Part model, mm, in its own coordinate system. A direction names the side the tool comes from. Round coordinates to 2 decimals unless told otherwise and drop trailing zeros. Order: outer loops, then holes, each group sorted by start corner. A loop starts at its lowest first (then second) coordinate and runs counter-clockwise, first axis right, second up. Notation, with made-up numbers: (66, 46) -> (114, 46) arc R29 ccw to (114, 78) -> close; hole circle Ø4 at (57, 71.5). An arc over 180 degrees is marked (long way). Answer as a JSON object with one key per item and string values. Group by question number.
```python
from build123d import *

# Parameters (mm, degrees)
SKETCH_5_R          = 3
EXTRUDE_4_DEPTH     = 5
CUT_EXTRUDE_2_DEPTH = 8.5
CUT_EXTRUDE_4_DEPTH = 8.5


with BuildPart() as part:
    # Sketch 5 → Extrude 4 (new body)
    with BuildSketch(Plane(origin=(0, 0, 0), x_dir=(1, 0, 0), z_dir=(0, 1, 0))):
        Polygon((-86.043555275, 72.404841583), (-103.043555275, 72.404841583), (-103.043555275, -36.501510282), (78.477843527, -36.501510282), (78.477843527, 72.404841583), (62.047530944, 72.404841583), (62.047530944, -18.742135335), (-86.043555275, -18.742135335), align=None)
        with BuildLine():
            ThreePointArc((-29.666312365, -34.509375465), (-31.566312365, -32.609375465), (-29.666312365, -30.709375465))
            Line((-29.666312365, -30.709375465), (-24.596682227, -30.709375465))
            ThreePointArc((-24.596682227, -30.709375465), (-22.696682227, -32.609375465), (-24.596682227, -34.509375465))
            Line((-24.596682227, -34.509375465), (-29.666312365, -34.509375465))
        make_face(mode=Mode.SUBTRACT)
        with BuildLine():
            ThreePointArc((0.233182571, -34.509375465), (-1.666817429, -32.609375465), (0.233182571, -30.709375465))
            Line((0.233182571, -30.709375465), (5.30281271, -30.709375465))
            ThreePointArc((5.30281271, -30.709375465), (7.20281271, -32.609375465), (5.30281271, -34.509375465))
            Line((5.30281271, -34.509375465), (0.233182571, -34.509375465))
        make_face(mode=Mode.SUBTRACT)
        with Locations(Location((-12.183568637, -27.595158417, 0), (0, 0, 270))):
            Circle(SKETCH_5_R, mode=Mode.SUBTRACT)
        with BuildLine():
            ThreePointArc((-29.666312365, -24.610941368), (-31.566842785, -22.710410948), (-29.666312365, -20.809880528))
            Line((-29.666312365, -20.809880528), (-24.596682227, -20.809880528))
            ThreePointArc((-24.596682227, -20.809880528), (-22.696151807, -22.710410948), (-24.596682227, -24.610941368))
            Line((-24.596682227, -24.610941368), (-29.666312365, -24.610941368))
        make_face(mode=Mode.SUBTRACT)
        with BuildLine():
            Line((0.233182571, -20.809880528), (5.30281271, -20.809880528))
            ThreePointArc((5.30281271, -20.809880528), (7.20281271, -22.709880528), (5.30281271, -24.609880528))
            Line((5.30281271, -24.609880528), (0.233182571, -24.609880528))
            ThreePointArc((0.233182571, -24.609880528), (-1.666817429, -22.709880528), (0.233182571, -20.809880528))
        make_face(mode=Mode.SUBTRACT)
    extrude(amount=EXTRUDE_4_DEPTH)

    # Sketch 5_14 → Cut-Extrude 2 (cut, symmetric)
    with BuildSketch(Plane(origin=(0, 0, 0), x_dir=(1, 0, 0), z_dir=(0, 1, 0))):
        with BuildLine():
            Line((-93.050173308, 59.6693943), (-93.050173308, 0))
            ThreePointArc((-93.050173308, 0), (-95.050173308, -2), (-97.050173308, 0))
            Line((-97.050173308, 0), (-97.050173308, 59.6693943))
            ThreePointArc((-97.050173308, 59.6693943), (-95.050173308, 61.6693943), (-93.050173308, 59.6693943))
        make_face()
    extrude(amount=CUT_EXTRUDE_2_DEPTH, both=True, mode=Mode.SUBTRACT)

    # Sketch 5_16 → Cut-Extrude 4 (cut, symmetric)
    with BuildSketch(Plane(origin=(0, 0, 0), x_dir=(1, 0, 0), z_dir=(0, 1, 0))):
        with BuildLine():
            Line((72.637966918, 59.6693943), (72.637966918, 0))
            ThreePointArc((72.637966918, 0), (70.637966918, -2), (68.637966918, 0))
            Line((68.637966918, 0), (68.637966918, 59.6693943))
            ThreePointArc((68.637966918, 59.6693943), (70.637966918, 61.6693943), (72.637966918, 59.6693943))
        make_face()
    extrude(amount=CUT_EXTRUDE_4_DEPTH, both=True, mode=Mode.SUBTRACT)


solid = part.part
```
Q1. Band-saw the part on C-C (x = 58). List the corners of the cut face in (y, z).
Q2. Band-saw the part on A-A (z = -19). List the corners of the cut face in (x, y).
Q3. Drop flat-ended pins along their axis: pin 1 Ø1 at (x, y) = (-29.5, 1) entering from -Z; pin 2 Ø5 at (x, z) = (-10, 16) entering from +Y. Give the stop position or say it passes through.
Q4. Which spindle directions (+Z, -Z, +X, -X, +Y, -Y) get a long thin tool onto all of the face, cutting with end or side? Do faces 4 (the cylindrical face through (-95.09, 2.54, -61.67)), 5 (the flat face through (-14, 2, 36.502)), 6 (the flat face through (62.048, 2, -27)). Say none if no direction does.
Q5. Two-plate mould, pull along Z, no slides. Class faces 1 (the flat face through (78.478, 2, -17)), 2 (the flat face through (-27, 2, 34.509)), 3 (the flat face through (70, 2, -72.405)): +Z half, -Z half, draft (parallel to the pull), parting line (faces both ways), or undercut.
Q6. Band-saw the part on B-B (y = 3.1). Count the separate pieces of the cut face and the enclosed holes in it, plus the area to 3 significant figures.
Q7. Wall check: line 1 (X direction, y = 1.15, z = -14.5); line 2 (Z direction, x = 0, y = 2.3); line 3 (X direction, y = 4.35, z = 4.5). Give the ranges that are in metal, low to high. Write a range as [from, to].
Completed:
{
 "1": {"outline": "(0, 18.74) -> (5, 18.74) -> (5, 36.5) -> (0, 36.5) -> close"},
 "2": {"outline": "(-103.04, 0) -> (-97.05, 0) -> (-97.05, 5) -> (-103.04, 5) -> close; (-93.05, 0) -> (-86.04, 0) -> (-86.04, 5) -> (-93.05, 5) -> close; (62.05, 0) -> (68.64, 0) -> (68.64, 5) -> (62.05, 5) -> close; (72.64, 0) -> (78.48, 0) -> (78.48, 5) -> (72.64, 5) -> close"},
 "3": {"pin 1": "z = 18.74", "pin 2": "through"},
 "4": {"face 4": "+Y, -Y", "face 5": "+Z, +X, -X, +Y, -Y", "face 6": "-Z, +Y, -Y"},
 "5": {"face 1": "draft", "face 2": "undercut", "face 3": "-Z half"},
 "6": {"separate pieces": "1", "enclosed holes": "7", "area": "5,620 mm2"},
 "7": {"line 1": "[-103.04, -97.05], [-93.05, -86.04], [62.05, 68.64], [72.64, 78.48]", "line 2": "[18.74, 20.82], [24.6, 30.72], [34.5, 36.5]", "line 3": "[-103.04, -86.04], [62.05, 78.48]"}
}
